from build123d import *

# Parameters (mm, degrees)
SKETCH_2_W          = 53.579793819
SKETCH_2_H          = 11.740278351
CUT_EXTRUDE_1_DEPTH = 64
SKETCH_3_W          = 57.586414551
SKETCH_3_H          = 11.064638604
SKETCH_3_W_2        = 48.61735144
SKETCH_3_H_2        = 9.555824249
CUT_EXTRUDE_2_DEPTH = 64
SKETCH_4_W          = 76
SKETCH_4_H          = 76
EXTRUDE_1_DEPTH     = 10
SKETCH_5_R          = 5
EXTRUDE_2_DEPTH     = 10


with BuildPart() as part:
    # 스케치1 → 회전1 (revolve)
    with BuildSketch(Plane.XY, mode=Mode.PRIVATE) as revolve_1_sk:
        Polygon((-16.680473815, 0), (-16.680473815, 30), (-5.680473815, 30), (-5.680473815, 21), (23.319526185, 21), (23.319526185, 17.5), (128.319526185, 17.5), (128.319526185, 0), align=None)
    revolve(revolve_1_sk.sketch.rotate(Axis((-16.680473815, 0, 0), (1, 0, 0)), 90), axis=Axis((-16.680473815, 0, 0), (1, 0, 0)))

    # 스케치2 → 컷-돌출1 (cut)
    with BuildSketch(Plane(origin=(128.319526185, 0, 0), x_dir=(0, 0, -1), z_dir=(1, 0, 0))):
        with Locations((8.115762888, 13.370139176)):
            Rectangle(SKETCH_2_W, SKETCH_2_H)
    extrude(amount=-CUT_EXTRUDE_1_DEPTH, mode=Mode.SUBTRACT)

    # 스케치3 → 컷-돌출2 (cut)
    with BuildSketch(Plane(origin=(-5.680473815, 0, 0), x_dir=(0, 0, -1), z_dir=(1, 0, 0))):
        with Locations((-0.377203588, 31.532319302)):
            Rectangle(SKETCH_3_W, SKETCH_3_H)
        with Locations((-1.173522276, -30.777912125)):
            Rectangle(SKETCH_3_W_2, SKETCH_3_H_2)
    extrude(amount=-CUT_EXTRUDE_2_DEPTH, mode=Mode.SUBTRACT)

    # 스케치4 → 보스-돌출1 (add)
    with BuildSketch(Plane.ZY.offset(16.680473815)):
        Rectangle(SKETCH_4_W, SKETCH_4_H)
    extrude(amount=EXTRUDE_1_DEPTH)

    # 스케치5 → 보스-돌출2 (add)
    with BuildSketch(Plane(origin=(0, 38, 0), x_dir=(1, 0, 0), z_dir=(0, 1, 0))):
        with BuildLine():
            ThreePointArc((-67.559960472, -12.763764728), (-74.680473815, 0), (-67.559960472, 12.763764728))
            Line((-67.559960472, 12.763764728), (-26.680473815, 38))
            Line((-26.680473815, 38), (-26.680473815, -38))
            Line((-26.680473815, -38), (-67.559960472, -12.763764728))
        make_face()
        with Locations(Location((-59.680473815, 0, 0), (0, 0, 270))):
            Circle(SKETCH_5_R, mode=Mode.SUBTRACT)
    extrude_2 = extrude(amount=-EXTRUDE_2_DEPTH)

    # 대칭 복사1: 보스-돌출2 across plane
    add(extrude_2.mirror(Plane.ZX))


solid = part.part
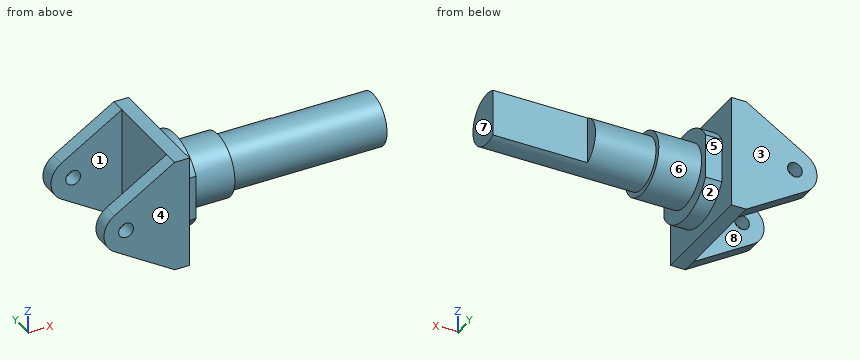
Can you work these out from the model? Positions are in its coordinate system, mm. Face numbers are marked on the shaded views. A direction names the side the tool comes from. Give positions to 0.01 mm unless a question says otherwise; leave off trailing zeros. Order: outer loops, then holes, each group sorted by start corner. A loop starts at its lowest first (then second) coordinate and runs counter-clockwise, first axis right, second up. Notation, with made-up numbers: M 50.5,70 L 93.5,70 A18 cw 93.5,87 Z; hole C -23.75,80.5 d1. An arc over 180 degrees is marked long. Use a Markdown table: item, result. Add a question column.
Item 1: Suppose I cut it at B-B (y = -5). List the corners of the cut face in (x, z) for me.
Item 2: Suppose I cut it at D-D (y = 31.5). List the corners of the cut face in (x, z) for me, then the cut area to 3 significant figures.
Item 3: Will these pins go through, and if not, where does the flat tip stop? pin 1 (12 mm diameter, centred on x = 2.5, y = 22.5, fed in from +Z); pin 2 (10 mm diameter, centred on x = 2.5, y = 22.5, fed in from -Z); pin 3 (1.5 mm diameter, centred on y = -27.5, z = -25, fed in from -X).
Item 4: Suppose I cut it at A-A (z = 0). Count the separate pieces of the cut face and the enclosed holes in it, then the cut area to 4 significant figures.
Item 5: We'd pull the mould along Y, two halves only. Please class the marked faces 1, 2, 3 and 4: +Y half, -Y half, draft (parallel to the pull), parting line (faces both ways), or undercut.
Item 6: If I drill on L1, parallel to X at y = 31.25, z = 0; L2, parallel to Y at x = -32.5, z = 25; L3, parallel to Z at x = 118, y = -9, over which ranges is the centre line in solid material (lowest first)? Write a range as [from, to].
Item 7: Suppose I cut it at C-C (z = -27). List the corners of the cut face in (x, y) for me.
Item 8: For the marked faces 5, 6, 7 and 8, which set-ups out of +Z, -Z, +X, -X, +Y, -Y let a thin tool reach every point of the face, with its end or its side?
Answer sheet:
| question | item | result |
|---|---|---|
| 1 | outline | M -26.68,-38 L -16.68,-38 L -16.68,-29.58 L -5.68,-29.58 L -5.68,-20.4 L 23.32,-20.4 L 23.32,-16.77 L 128.32,-16.77 L 128.32,16.77 L 23.32,16.77 L 23.32,20.4 L -5.68,20.4 L -5.68,29.58 L -16.68,29.58 L -16.68,38 L -26.68,38 Z |
| 2 | outline | M -67.56,-12.76 L -26.68,-38 L -16.68,-38 L -16.68,38 L -26.68,38 L -67.56,12.76 A15 ccw Z; hole C -59.68,0 d10 |
| 2 | area | 2,890 mm² |
| 3 | pin 1 | stops at z = 12.99 |
| 3 | pin 2 | stops at z = -11.61 |
| 3 | pin 3 | stops at x = -48.64 |
| 4 | separate pieces | 3 |
| 4 | enclosed holes | 0 |
| 4 | area | 6,345 mm² |
| 5 | face 1 | undercut |
| 5 | face 2 | parting line |
| 5 | face 3 | +Y half |
| 5 | face 4 | -Y half |
| 6 | L1 | x = [-74.68, -64.68], [-54.68, -16.68] |
| 6 | L2 | y = [-38, -28], [28, 38] |
| 6 | L3 | z = [-15.01, 15.01] |
| 7 | outline | M -44.5,-38 L -16.68,-38 L -16.68,-13.08 L -5.68,-13.08 L -5.68,13.08 L -16.68,13.08 L -16.68,38 L -44.5,38 L -44.5,28 L -26.68,28 L -26.68,-28 L -44.5,-28 Z |
| 8 | face 5 | +Z, -Z, +X, +Y |
| 8 | face 6 | +X |
| 8 | face 7 | +Z, -Z, +X, +Y, -Y |
| 8 | face 8 | +Z, -Z, -X |
